The model under review builds one solid part; all positions refer to its coordinate system, in mm. A direction names the side the tool comes from. Round coordinates to 2 decimals unless told otherwise and drop trailing zeros. Write each loop counter-clockwise with the first axis right and the second up, starting at its lowest first coordinate (ties: lowest second). Pieces come first, ordered by that corner, then holes. Notation, with made-up numbers: M 56.25,14 L 76.25,14 A26 cw 76.25,36 Z; hole C -36,69.25 d8. An arc over 180 degrees is marked long. Write item = value, one per line. Start each with the question number.
Item 1: To check wall thickness, follow line 1 along Y through (x, z) = (0, -0.35) (3 decimals); line 2 along Z through (x, y) = (5.75, -6.5); line 3 along Z through (x, y) = (-10, 7.75). State the ranges of each line that lie inside material, in increasing order.
Item 2: Tool access review of faces 1 (the flat face through (-9, -1.587, 11)), 2 (the flat face through (-1.587, 9, 11)), 3 (the flat face through (7, -7, 20.312)): name each direction out of +Z, -Z, +X, -X, +Y, -Y from which nothing blocks a thin tool from reaching the whole face with its end or side.
Item 3: Take a section at A-A, the plane y = 0. Give the boundary of the cut face in (x, z) (1 decimal).
Item 4: For pin 1 Ø5.5 at (x, y) = (5.5, 8.5) entering from -Z; pin 2 Ø3 at (x, z) = (-10, 9) entering from +Y; pin 3 Ø5 at (y, z) = (-10.5, 12) entering from +X, all flat-tipped, find the tip position at first contact; note any pin that passes through.
Item 5: The part is to be moulded in two halves that separate along Z. For faces 4 (the flat face through (-1.588, -9, 11)), 5 (the flat face through (5, -9, -0.794)), 6 (the cylindrical face through (-7.137, -0.314, -1.612)), 7 (the flat face through (4, -2, 21.899)), say which applies: +Z half, -Z half, draft (parallel to the pull), parting line (faces both ways), or undercut.
Item 6: Take a section at D-D, the plane y = 10.5. Give the boundary of the cut face in (x, z), plus the area to 3 significant figures.
Item 7: Take a section at C-C, the plane z = -2. Give the boundary of the cut face in (x, y), plus the area to 3 significant figures.
from build123d import *

# Parameters (mm, degrees)
F0_R             = 12.7
F0_R_2           = 3.96875
F1_DEPTH         = 1.5875
F2_R             = 12.7
F2_R_2           = 9.525
F3_DEPTH         = 0.79375
F4_R             = 6.35
F4_R_2           = 3.96875
F5_DEPTH         = 18.7244736
F6_R             = 12.7
F6_R_2           = 3.96875
F7_DEPTH         = 1.5875
F8_R             = 12.7
F8_R_2           = 9.525
F9_DEPTH         = 0.79375
F11_DEPTH        = 18.7244736
F11_COPIES_COUNT = 4
F12_R            = 7.14375
F12_R_2          = 3.96875
F13_DEPTH        = 4.85775
F14_SIZE         = 1.5875


# Not quite as in the source:
# - a length typed as a fraction of an inch, garbled in the dataset ("3 / 203.2 mm" for 3/8 in), is restored
# - a pattern or mirror of a feature is missing from the dataset's text; its kind, count and spacing are read off the source's solid


with BuildPart() as f1:
    # F0 (on Top) → F1 (new body)
    with BuildSketch(Plane.XY):
        Circle(F0_R)
        Circle(F0_R_2, mode=Mode.SUBTRACT)
    extrude(amount=F1_DEPTH)

    # F2 (on face) → F3 (join)
    with BuildSketch(Plane(origin=(0, 0, 0), x_dir=(1, 0, 0), z_dir=(0, 0, -1))):
        Circle(F2_R)
        Circle(F2_R_2, mode=Mode.SUBTRACT)
    extrude(amount=F3_DEPTH)

    # F4 (on face) → F5 (join)
    with BuildSketch(Plane.XY.offset(1.5875)):
        Circle(F4_R)
        Circle(F4_R_2, mode=Mode.SUBTRACT)
    extrude(amount=F5_DEPTH)

    # F6 (on face) → F7 (join)
    with BuildSketch(Plane.XY.offset(20.3119736)):
        Circle(F6_R)
        Circle(F6_R_2, mode=Mode.SUBTRACT)
    extrude(amount=F7_DEPTH)

    # F8 (on face) → F9 (join)
    with BuildSketch(Plane.XY.offset(21.8994736)):
        Circle(F8_R)
        Circle(F8_R_2, mode=Mode.SUBTRACT)
    extrude(amount=F9_DEPTH)

    # F10 (on face) → F11 (join, through all)
    with BuildSketch(Plane.XY.offset(1.5875)):
        with BuildLine():
            Line((1.5875, -12.6003906189), (1.5875, -6.1483610621))
            ThreePointArc((1.5875, -6.1483610621), (0, -6.35), (-1.5875, -6.1483610621))
            Line((-1.5875, -6.1483610621), (-1.5875, -12.6003906189))
            ThreePointArc((-1.5875, -12.6003906189), (0, -12.7), (1.5875, -12.6003906189))
        make_face()
    f11 = extrude(amount=F11_DEPTH)

    # F11_copies: F11 ×4 about axis
    f11_copies_axis = Axis((0, 0, 0), (0, 0, 1))
    for i in range(1, F11_COPIES_COUNT):
        add(f11.rotate(f11_copies_axis, i * 360 / F11_COPIES_COUNT))

    # F12 (on face) → F13 (join)
    with BuildSketch(Plane(origin=(0, 0, 0), x_dir=(1, 0, 0), z_dir=(0, 0, -1))):
        Circle(F12_R)
        Circle(F12_R_2, mode=Mode.SUBTRACT)
    extrude(amount=F13_DEPTH)

    # F14
    f14_edges = [f1.edges().sort_by_distance(p)[0] for p in [
        (-7.14375, 0, -4.85775),
    ]]
    chamfer(f14_edges, length=F14_SIZE)


solid = f1.part
Response values:
q1.line_1 = -12.7 to -9.525, -7.144 to -3.969, 3.969 to 7.144, 9.525 to 12.7
q1.line_2 = 0 to 1.59, 20.31 to 21.9
q1.line_3 = -0.79 to 1.59, 20.31 to 22.69
q2.face_1 = -X, -Y
q2.face_2 = -X, +Y
q2.face_3 = +X, -Y
q3.outline = M -12.7,-0.8 L -9.5,-0.8 L -9.5,0 L -7.1,0 L -7.1,-3.3 L -5.6,-4.9 L -4,-4.9 L -4,21.9 L -9.5,21.9 L -9.5,22.7 L -12.7,22.7 Z; M 4,-4.9 L 5.6,-4.9 L 7.1,-3.3 L 7.1,0 L 9.5,0 L 9.5,-0.8 L 12.7,-0.8 L 12.7,22.7 L 9.5,22.7 L 9.5,21.9 L 4,21.9 Z
q4.pin_1 = -0.79
q4.pin_2 = 1.59
q4.pin_3 = 1.59
q5.face_4 = undercut
q5.face_5 = -Z half
q5.face_6 = draft
q5.face_7 = +Z half
q6.outline = M -7.14,-0.79 L 7.14,-0.79 L 7.14,1.59 L 1.59,1.59 L 1.59,20.31 L 7.14,20.31 L 7.14,22.69 L -7.14,22.69 L -7.14,20.31 L -1.59,20.31 L -1.59,1.59 L -7.14,1.59 Z
q6.area = 127 mm2
q7.outline = C 0,0 d14.29; hole C 0,0 d7.94
q7.area = 111 mm2
